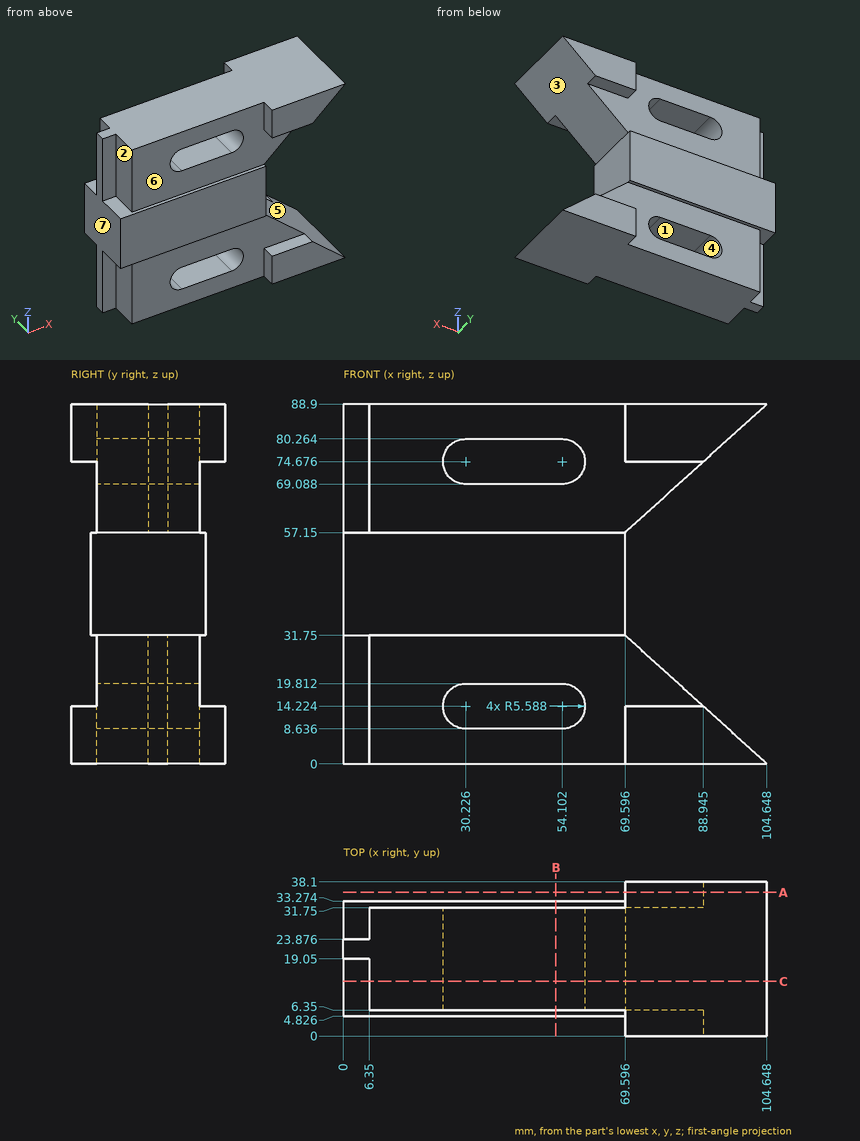
Can you work these out from the drawing? Everything is in mm from the part's minimum corner. A direction names the side the tool comes from. Give positions to 0.01 mm unless a question says otherwise; leave off trailing zeros. Order: outer loops, then holes, each group sorted by start corner. A loop starts at its lowest first (then second) coordinate and runs counter-clockwise, first axis right, second up. Notation, with made-up numbers: M 38.25,36 L 50.25,36 A8 ccw 50.25,40 Z; hole C 14.25,55 d9. An arc over 180 degrees is marked long. Use a Markdown table: item, result. Add a question column.
1. Suppose I cut it at A-A (y = 35.5). List the corners of the cut face in (x, z) for me (1 decimal).
2. On a 3-axis mill with a long thin cutter (end or side, diameter ignored), from which of +Z, -Z, +X, -X, +Y, -Y can I reach the whole of each face in a straight line? I mean the marked faces 1, 2 and 3. Say none if no direction works.
3. Suppose I cut it at C-C (y = 13.5). List the corners of the cut face in (x, z) for me, and give its area (3 significant figures).
4. Suppose I cut it at B-B (x = 52.5). List the corners of the cut face in (y, z) for me, and give its area (3 significant figures).
5. If we mould it in two halves opening along X, with no side actions, what happens to the marked faces 4, 5, 6 and 7? For each: +X half, -X half, draft (parallel to the pull), parting line (faces both ways), or undercut.
6. I need wall thicknesses on probe 1 along Z at (x, y) = (42.5, 27); probe 2 along Z at (x, y) = (57, 30) (1 decimal); probe 3 along Z at (x, y) = (87, 3). Which ranges of each line are inside material? Lowest first, please. Write a range as from..to.
7. For pin 1 Ø10 at (y, z) = (18, 66.5) entering from +X; pin 2 Ø5 at (x, z) = (3, 74.5) entering from -Y; pin 3 Ø12.5 at (x, z) = (48.5, 40.5) entering from +Y; pin 4 Ø6 at (x, y) = (20, 16.5) entering from -Z, each with a flat end and sliding along its axis, tell me the tip position at first contact or that it passes through.
Results list:
| question | item | result |
|---|---|---|
| 1 | outline | M 69.6,0 L 104.6,0 L 88.9,14.2 L 69.6,14.2 Z; M 69.6,74.7 L 88.9,74.7 L 104.6,88.9 L 69.6,88.9 Z |
| 2 | face 1 | +Y, -Y |
| 2 | face 2 | +Z, -X, -Y |
| 2 | face 3 | +X, +Y, -Y |
| 3 | outline | M 0,31.75 L 6.35,31.75 L 6.35,0 L 104.65,0 L 69.6,31.75 L 69.6,57.15 L 104.65,88.9 L 6.35,88.9 L 6.35,57.15 L 0,57.15 Z; hole M 30.23,8.64 L 54.1,8.64 A5.59 ccw 54.1,19.81 L 30.23,19.81 A5.59 ccw Z; hole M 30.23,69.09 L 54.1,69.09 A5.59 ccw 54.1,80.26 L 30.23,80.26 A5.59 ccw Z |
| 3 | area | 6,170 mm² |
| 4 | outline | M 4.83,31.75 L 6.35,31.75 L 6.35,19.81 L 31.75,19.81 L 31.75,31.75 L 33.27,31.75 L 33.27,57.15 L 31.75,57.15 L 31.75,69.09 L 6.35,69.09 L 6.35,57.15 L 4.83,57.15 Z; M 6.35,0 L 31.75,0 L 31.75,8.64 L 6.35,8.64 Z; M 6.35,80.26 L 31.75,80.26 L 31.75,88.9 L 6.35,88.9 Z |
| 4 | area | 1,770 mm² |
| 5 | face 4 | undercut |
| 5 | face 5 | +X half |
| 5 | face 6 | draft |
| 5 | face 7 | -X half |
| 6 | probe 1 | z = 0..8.64, 19.81..69.09, 80.26..88.9 |
| 6 | probe 2 | z = 0..9.4, 19..69.9, 79.5..88.9 |
| 6 | probe 3 | z = 0..14.22, 74.68..88.9 |
| 7 | pin 1 | stops at x = 85.44 |
| 7 | pin 2 | stops at y = 19.05 |
| 7 | pin 3 | stops at y = 33.27 |
| 7 | pin 4 | stops at z = 0 |
